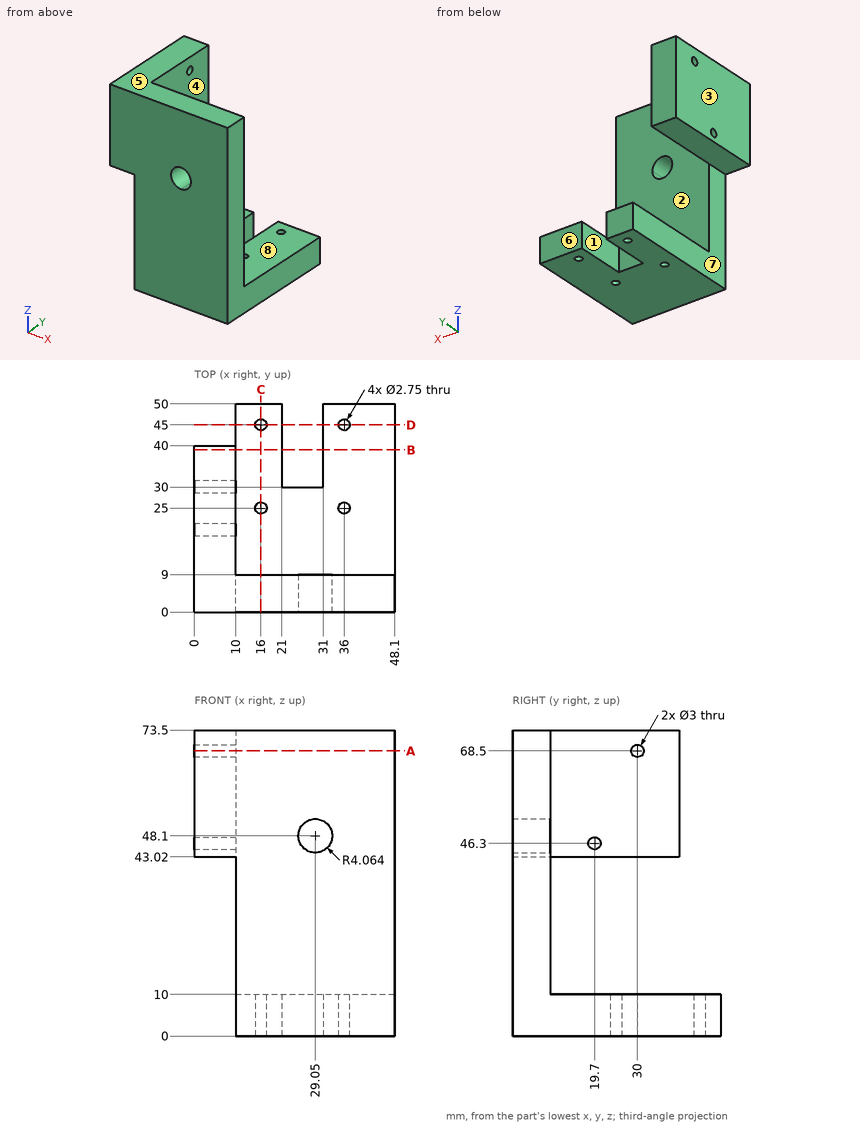
Study the drawing (mm; zero at the part's minimum x, y, z) and answer. A direction names the side the tool comes from. Coordinates: 2 decimals unless noted, no trailing zeros. Order: outer loops, then holes, each group sorted by start corner. A loop starts at its lowest first (then second) coordinate and runs counter-clockwise, first axis right, second up. Notation, with made-up numbers: (71, 69.25) -> (103, 69.25) arc R24 cw to (103, 82.25) -> close; hole circle Ø6 at (45, 35). An arc over 180 degrees is marked (long way). Answer in a Markdown table with one row per item. Add a question column.
Item 1: Find section D-D (y = 45). Write down the section's boundary in (x, z) (3 decimals).
Item 2: Find section A-A (z = 68.5). Write down the section's boundary in (x, y), then the cut area to 3 significant figures.
Item 3: Find section B-B (y = 39). Write down the section's boundary in (x, z).
Item 4: Determine the mould class of the marked faces 1, 2 and 3 for opening direction X: +X half, -X half, draft (parallel to the pull), parting line (faces both ways), or undercut.
Item 5: Which of the six approach directions +Z, -Z, +X, -X, +Y, -Y give full straight-line access (tool end or side, diameter ignored) to the marked faces 4, 5, 6, 7 and 8?
Item 6: Find the intervals of material crossed by L1, parallel to Y at x = 16, z = 4.25 (3 decimals); L2, parallel to Y at x = 2.75, z = 46.3; L3, parallel to Z at x = 6.5, y = 11, in increasing order. Write a range as from..to.
Item 7: Each of these flat-tipped pins is pushed along its axis until it touches: P1, Ø24.5, axis at y = 22.5, z = 62, coming from the +X side; P2, Ø21.5, axis at y = 15, z = 17.5, coming from the -X side; P3, Ø2, axis at x = 16, y = 45, coming from the -Z side; P4, Ø12, axis at x = 41, y = 40, coming from the +Z side. Where does it stop, or does it pass through?
Item 8: Find section C-C (x = 16). Write down the section's boundary in (y, z) (3 decimals).
Result set:
| question | item | result |
|---|---|---|
| 1 | outline | (10, 0) -> (14.625, 0) -> (14.625, 10) -> (10, 10) -> close; (17.375, 0) -> (21, 0) -> (21, 10) -> (17.375, 10) -> close; (31, 0) -> (34.625, 0) -> (34.625, 10) -> (31, 10) -> close; (37.375, 0) -> (48.1, 0) -> (48.1, 10) -> (37.375, 10) -> close |
| 2 | outline | (0, 0) -> (48.1, 0) -> (48.1, 9) -> (10, 9) -> (10, 28.5) -> (0, 28.5) -> close; (0, 31.5) -> (10, 31.5) -> (10, 40) -> (0, 40) -> close |
| 2 | area | 713 mm² |
| 3 | outline | (0, 43.02) -> (10, 43.02) -> (10, 73.5) -> (0, 73.5) -> close; (10, 0) -> (21, 0) -> (21, 10) -> (10, 10) -> close; (31, 0) -> (48.1, 0) -> (48.1, 10) -> (31, 10) -> close |
| 4 | face 1 | undercut |
| 4 | face 2 | draft |
| 4 | face 3 | -X half |
| 5 | face 4 | +Z, +X, +Y |
| 5 | face 5 | +Z, +X, -X, +Y, -Y |
| 5 | face 6 | +Z, -Z, +X, -X, +Y |
| 5 | face 7 | -Z, -X, +Y, -Y |
| 5 | face 8 | +Z, +X, -X, +Y |
| 6 | L1 | y = 0..23.625, 26.375..43.625, 46.375..50 |
| 6 | L2 | y = 0..18.2, 21.2..40 |
| 6 | L3 | z = 43.02..73.5 |
| 7 | P1 | stops at x = 10 |
| 7 | P2 | stops at x = 10 |
| 7 | P3 | passes through |
| 7 | P4 | stops at z = 10 |
| 8 | outline | (0, 0) -> (23.625, 0) -> (23.625, 10) -> (9, 10) -> (9, 73.5) -> (0, 73.5) -> close; (26.375, 0) -> (43.625, 0) -> (43.625, 10) -> (26.375, 10) -> close; (46.375, 0) -> (50, 0) -> (50, 10) -> (46.375, 10) -> close |
